Model file for the job. Use its own axes, mm. A direction names the side the tool comes from. Coordinates: 2 decimals unless noted, no trailing zeros. Loops run counter-clockwise (first coordinate to the right, second up) from the corner with the lowest first, then second, coordinate; pieces in that order, holes last.
from build123d import *

# Parameters (mm, degrees)
CUT_EXTRUDE1_DEPTH      = 5.816666667
CUT_EXTRUDE1_DEPTH_BACK = 10
SKETCH3_R               = 2.75
CUT_EXTRUDE2_DEPTH      = 3.0000001
CUT_EXTRUDE2_DEPTH_BACK = 7.0000001


with BuildPart() as part:
    # Sketch1 → Revolve1 (revolve)
    with BuildSketch(Plane.XY):
        with BuildLine():
            Line((0, 0), (0, 56))
            Line((0, 56), (-2, 56))
            Line((-2, 56), (-2, 0))
            Line((-2, 0), (-4, 0))
            Line((-4, 0), (-4, -11.5))
            ThreePointArc((-4, -11.5), (-4.25, -16.45), (0, -19))
            Line((0, -19), (0, 0))
        make_face()
    revolve(axis=Axis((0, 0, 0), (0, 1, 0)))

    # Sketch2 → Cut-Extrude1 (cut, two sides)
    with BuildSketch(Plane(origin=(0, 0, 0), x_dir=(0, 0, -1), z_dir=(1, 0, 0))) as cut_extrude1_sk:
        with BuildLine():
            ThreePointArc((-2, -8.5), (-2.881966011, -7.763932023), (-4, -7.5))
            Line((-4, -7.5), (-4, -8.077978136))
            ThreePointArc((-4, -8.077978136), (-6.041123222, -13.901532194), (-2, -18.56514549))
            Line((-2, -18.56514549), (-2, -11.5))
            Line((-2, -11.5), (-2, -8.5))
        make_face()
        with BuildLine():
            Line((4, -8.077978136), (4, -7.5))
            ThreePointArc((4, -7.5), (2.881966011, -7.763932023), (2, -8.5))
            Line((2, -8.5), (2, -11.5))
            Line((2, -11.5), (2, -18.56514549))
            ThreePointArc((2, -18.56514549), (6.041123222, -13.901532194), (4, -8.077978136))
        make_face()
    extrude(amount=CUT_EXTRUDE1_DEPTH, mode=Mode.SUBTRACT)
    extrude(cut_extrude1_sk.sketch, amount=-CUT_EXTRUDE1_DEPTH_BACK, mode=Mode.SUBTRACT)

    # Sketch3 → Cut-Extrude2 (cut, two sides)
    with BuildSketch(Plane.XY.offset(2)) as cut_extrude2_sk:
        with Locations((0, -14)):
            Circle(SKETCH3_R)
    extrude(amount=CUT_EXTRUDE2_DEPTH, mode=Mode.SUBTRACT)
    extrude(cut_extrude2_sk.sketch, amount=-CUT_EXTRUDE2_DEPTH_BACK, mode=Mode.SUBTRACT)


solid = part.part
Q1. Which spindle directions (+Z, -Z, +X, -X, +Y, -Y) get a long thin tool onto all of the face, cutting with end or side? Do faces 4 (the flat face through (-1, -11, 2)), 5 (the flat face through (0, 56, 0)), 6 (the cylindrical face through (0, 28, -2)), 7 (the flat face through (0, -11, -2)). Say none if no direction does.
Answers:
face 4: +Z, +X, -X, -Y
face 5: +Z, -Z, +X, -X, +Y
face 6: +Y
face 7: -Z, +X, -X, -Y
Q2. Slice it at B-B (z = 0). List the corners of the cut face in (x, y).
Answers:
outline: (-4, -11.5) arc R4.82 ccw (long way) to (4, -11.5) - (4, 0) - (2, 0) - (2, 56) - (-2, 56) - (-2, 0) - (-4, 0) - close; hole circle Ø5.5 at (0, -14)
Q3. Slice it at A-A (x = 0). List the corners of the cut face in (y, z), and give its area (3 significant figures).
Answers:
outline: (-18.57, -2) - (-16.75, -2) - (-16.75, 2) - (-18.57, 2) arc R4.82 ccw to start; (-11.25, -2) - (-8.5, -2) arc R2.5 cw to (-7.5, -4) - (0, -4) - (0, -2) - (56, -2) - (56, 2) - (0, 2) - (0, 4) - (-7.5, 4) arc R2.5 cw to (-8.5, 2) - (-11.25, 2) - close
area: 309 mm2
Q4. Drill centre lines: line 1 (Y direction, x = 0, z = -0.35); line 2 (Y direction, x = -2.5, z = 0.5); line 3 (X direction, y = 14.5, z = -0.25). Where is each one in solid material? Low to high.
Answers:
line 1: y = -18.99 to -16.75, -11.25 to 56
line 2: y = -18.27 to -15.15, -12.85 to 0
line 3: x = -1.98 to 1.98
Q5. Mould opens along X. For faces 1 (the cylindrical face through (-3.695, -4.553, -1.532)), 2 (the cylindrical face through (-0.358, -11.273, 0.028)), 3 (the cylindrical face through (-0.048, -7.882, -2.672)) say: +X half, -X half, draft (parallel to the pull), parting line (faces both ways), or undercut.
Answers:
face 1: parting line
face 2: undercut
face 3: draft
Q6. Flat gauge pins, fed straight in: P1, Ø3, axis at x = -2.5, y = -7.5, coming from the -Z side; P2, Ø4.5, axis at x = 0.5, y = -11.5, coming from the -Z side; P3, Ø2, axis at x = 3.5, z = -0.5, coming from the -Y side. Where does each tip first touch, or does it go through?
Answers:
P1: stops at z = -3.87
P2: stops at z = -2
P3: stops at y = -18.28
Q7. Slice it at C-C (y = -14). List the corners of the cut face in (x, z).
Answers:
outline: (-4.38, -2) - (-2.75, -2) - (-2.75, 2) - (-4.38, 2) arc R4.81 ccw to start; (2.75, -2) - (4.38, -2) arc R4.81 ccw to (4.38, 2) - (2.75, 2) - close
Q8. Slice it at D-D (y = 37). List the corners of the cut face in (x, z), and give its area (3 significant figures).
Answers:
outline: circle Ø4 at (0, 0)
area: 12.6 mm2
